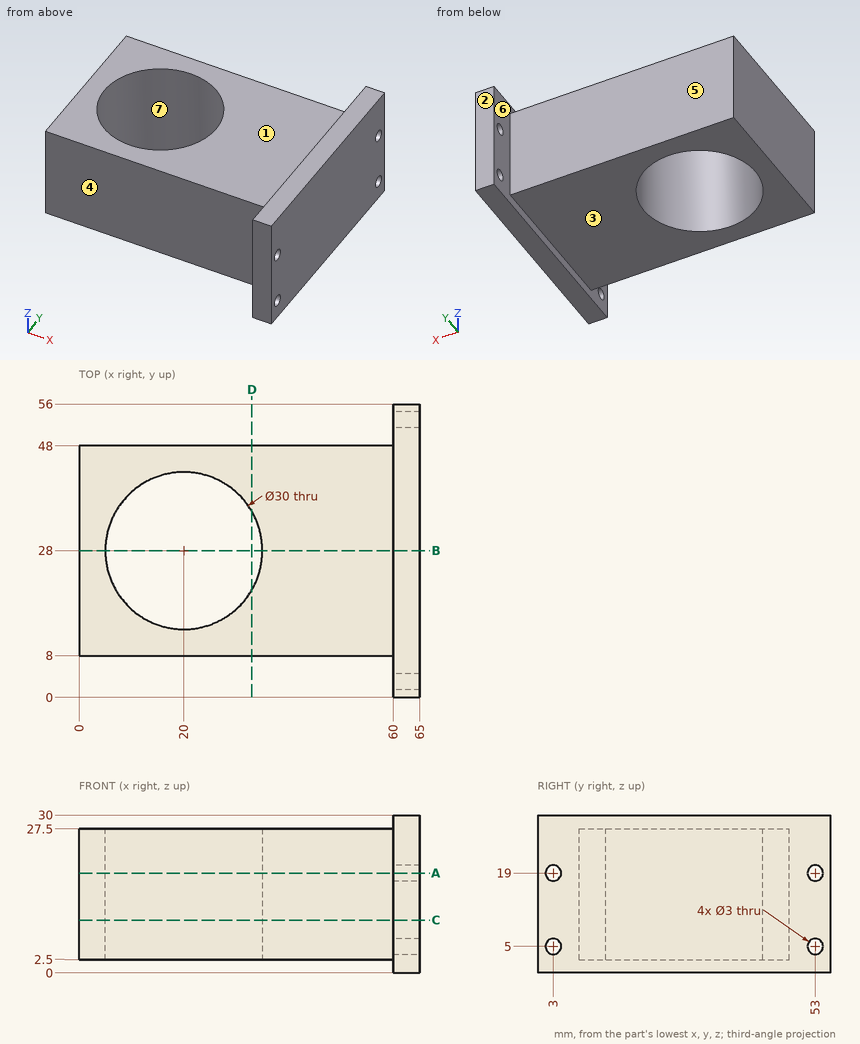
Study the drawing (mm; zero at the part's minimum x, y, z) and answer. A direction names the side the tool comes from. Coordinates: 2 decimals unless noted, no trailing zeros. Order: outer loops, then holes, each group sorted by start corner. A loop starts at its lowest first (then second) coordinate and runs counter-clockwise, first axis right, second up. Notation, with made-up numbers: M 67,36 L 112,36 A21 cw 112,62 Z; hole C 16.25,30 d4. An arc over 180 degrees is marked long. Use CSV: the item, a comma, the result in double quotes.
Q1. Section D-D (x = 33) is taken. Determine the outline of the cut face in (y, z), then the cut area to 3 significant figures.
Here are the results:
outline,"M 8,2.5 L 20.52,2.5 L 20.52,27.5 L 8,27.5 Z; M 35.48,2.5 L 48,2.5 L 48,27.5 L 35.48,27.5 Z"
area,"626 mm2"
Q2. Straight lines are drawn through the part: L1, parallel to Y at x = 62, z = 19; L2, parallel to X at y = 53, z = 22.5; L3, parallel to Y at x = 31, z = 21. For each, find the intervals that lie inside material, in ascending order.
Here are the results:
L1,"0 to 1.5, 4.5 to 51.5, 54.5 to 56"
L2,"60 to 65"
L3,"8 to 17.8, 38.2 to 48"
Q3. Section A-A (z = 19) is taken. Determine the outline of the cut face in (x, y), then the cut area to 3 significant figures.
Here are the results:
outline,"M 0,8 L 60,8 L 60,4.5 L 65,4.5 L 65,51.5 L 60,51.5 L 60,48 L 0,48 Z; M 60,0 L 65,0 L 65,1.5 L 60,1.5 Z; M 60,54.5 L 65,54.5 L 65,56 L 60,56 Z; hole C 20,28 d30"
area,"1,940 mm2"
Q4. A tool of negligible diameter and unlimited length cuts with its end or side. For the marked faces 1, 2, 3 and 4, from which of +Z, -Z, +X, -X, +Y, -Y can it reach the whole face along a straight path? Write none if from no direction.
Here are the results:
face 1,"+Z, -X, +Y, -Y"
face 2,"+Z, -Z, +X, -X, +Y"
face 3,"-Z, -X, +Y, -Y"
face 4,"+Z, -Z, -X, -Y"
Q5. Section B-B (y = 28) is taken. Determine the outline of the cut face in (x, z).
Here are the results:
outline,"M 0,2.5 L 5,2.5 L 5,27.5 L 0,27.5 Z; M 35,2.5 L 60,2.5 L 60,0 L 65,0 L 65,30 L 60,30 L 60,27.5 L 35,27.5 Z"
Q6. Section C-C (z = 10) is taken. Determine the outline of the cut face in (x, y).
Here are the results:
outline,"M 0,8 L 60,8 L 60,0 L 65,0 L 65,56 L 60,56 L 60,48 L 0,48 Z; hole C 20,28 d30"
Q7. Given pin 1 Ø8 at (x, z) = (23.5, 22.5) entering from -Y; pin 2 Ø12 at (x, y) = (44.5, 45) entering from -Z; pin 3 Ø5 at (y, z) = (21.5, 8.5) entering from -X; pin 4 Ø2 at (x, y) = (50, 35) entering from +Z, each flat-ended and moving along its own axis, determine where each tip first touches the part or whether it passes through.
Here are the results:
pin 1,"y = 8"
pin 2,"z = 2.5"
pin 3,"x = 0"
pin 4,"z = 27.5"
Q8. Determine the mould class of the marked faces 5, 6 and 7 for opening direction Y: pulls with the +Y half, pulls with the -Y half, needs draft (parallel to the pull), parting line crosses it, or undercut.
Here are the results:
face 5,"pulls with the +Y half"
face 6,"needs draft"
face 7,"undercut"
